For this review, take the finished solid that the model builds, in its own axes (mm). Face numbers are marked on the shaded views. A direction names the side the tool comes from. Give positions to 0.01 mm unless a question says otherwise; leave off trailing zeros. Loops run counter-clockwise (first coordinate to the right, second up) from the corner with the lowest first, then second, coordinate; pieces in that order, holes last. Notation, with made-up numbers: (23.25, 33) - (78.25, 33) arc R34 cw to (78.25, 71) - close; hole circle Ø3 at (56.5, 80.25). An arc over 180 degrees is marked (long way). Answer as CSV lines item,"result".
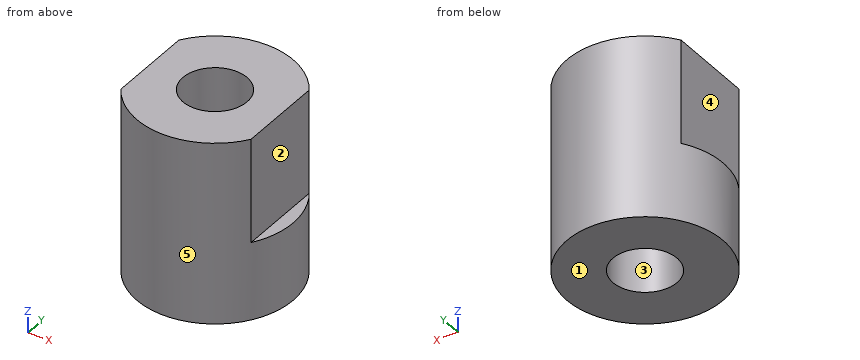
Autodesk Inventor part; units mm, degrees
ref_plane "YZ Plane" through (0, 0, 0) normal (1, 0, 0) x (0, 1, 0)
ref_plane "XZ Plane" through (0, 0, 0) normal (0, 1, 0) x (-1, 0, 0)
ref_plane "XY Plane" through (0, 0, 0) normal (0, 0, 1) x (1, 0, 0)
sketch "Sketch1" plane through (0, 0, 0) normal (0, 0, 1) x (1, 0, 0)
  circle A0 centre (0, 0) radius 3
  dimension "d0" = 6
extrude "Extrusion1" add sketch "Sketch1" along normal blind 7
sketch "Sketch2" plane through (0, 0, 7) normal (0, 0, 1) x (1, 0, 0)
  point P0 (0, 0)
  point P1 (0, 0)
hole "Hole1" at (0, 0, 7) direction (0, 0, -1) diameter 2.459 end through all
sketch "Sketch3" plane through (0, 0, 0) normal (0, 1, 0) x (-1, 0, 0)
  line L0 (3, 0) -> (3, 7)
  line L1 (3, 7) -> (2.5, 7)
  line L2 (2.5, 7) -> (2.5, 3)
  line L3 (2.5, 3) -> (3, 3)
  line L4 (3, 3) -> (3, 7)
  line L5 (3, 7) -> (-3, 7)
  line L6 (-3, 7) -> (-2.5, 7)
  line L7 (-2.5, 7) -> (-2.5, 3)
  line L8 (-2.5, 3) -> (-3, 3)
  line L9 (-3, 3) -> (-3, 7)
  point P0 (0, 0)
  dimension "d10" = 0.5
  dimension "d11" = 5
  dimension "d12" = 0.5
  dimension "d13" = 4
extrude "Extrusion2" cut sketch "Sketch3" along normal through all both and the other way through all
equation "\"d10\" = d12"
properties part number "Timing_Lever Weight" material "Aluminum 6061"
1) Machinability: for the marked faces 4 and 5, which of the approach directions +Z, -Z, +X, -X, +Y, -Y give a long, thin tool a straight path to every point of the face, cutting with its end or side? Answer none if there is none.
From the geometry:
face 4,"+Z, -X, +Y, -Y"
face 5,"+Z, -Z"
2) Wall thickness on line 1 (X direction, y = 0, z = 4); line 2 (Y direction, x = 0, z = 5); line 3 (X direction, y = 0.35, z = 2.5): over which ranges is each line inside the solid? List them lowest first. Write a range as from..to.
From the geometry:
line 1,"x = -2.5..-1.23, 1.23..2.5"
line 2,"y = -3..-1.23, 1.23..3"
line 3,"x = -2.98..-1.18, 1.18..2.98"
3) Insertion check: P1, Ø1.5, axis at y = -1.5, z = 5, coming from the -X side; P2, Ø1, axis at x = -1, z = 5.5, coming from the +Y side; P3, Ø2, axis at x = 1.5, z = 4, coming from the -Y side. Each pin has a flat end and moves straight along its axis. Give the tip position at first contact, or say it passes through.
From the geometry:
P1,"stops at x = -2.5"
P2,"stops at y = 2.96"
P3,"stops at y = -2.96"
4) Consider section D-D on y = -0.85. Write out the cut boundary in (x, z), and give its area (3 significant figures).
From the geometry:
outline,"(-2.88, 0) - (-0.89, 0) - (-0.89, 7) - (-2.5, 7) - (-2.5, 3) - (-2.88, 3) - close; (0.89, 0) - (2.88, 0) - (2.88, 3) - (2.5, 3) - (2.5, 7) - (0.89, 7) - close"
area,"24.8 mm^2"
5) Draft analysis for pull direction X (two halves, no side actions). For the marked faces 1, 2 and 3, state which applies: pulls with the +X half, pulls with the -X half, needs draft (parallel to the pull), parting line crosses it, or undercut.
From the geometry:
face 1,"needs draft"
face 2,"pulls with the +X half"
face 3,"undercut"
6) Consider section A-A on y = 0. Write out the cut boundary in (x, z).
From the geometry:
outline,"(-3, 0) - (-1.23, 0) - (-1.23, 7) - (-2.5, 7) - (-2.5, 3) - (-3, 3) - close; (1.23, 0) - (3, 0) - (3, 3) - (2.5, 3) - (2.5, 7) - (1.23, 7) - close"
7) Consider section C-C on z = 3.5. Write out the cut boundary in (x, y), and give its area (3 significant figures).
From the geometry:
outline,"(-2.5, -1.66) arc R3 ccw to (2.5, -1.66) - (2.5, 1.66) arc R3 ccw to (-2.5, 1.66) - close; hole circle Ø2.46 at (0, 0)"
area,"21.3 mm^2"
8) Consider section B-B on x = 0.3. Write out the cut boundary in (y, z), and give its area (3 significant figures).
From the geometry:
outline,"(-2.98, 0) - (-1.19, 0) - (-1.19, 7) - (-2.98, 7) - close; (1.19, 0) - (2.98, 0) - (2.98, 7) - (1.19, 7) - close"
area,"25.1 mm^2"
